Can you work these out from the model? Positions are in its coordinate system, mm. Give positions to 0.01 mm unless a question says otherwise; leave off trailing zeros. Order: outer loops, then holes, each group sorted by start corner. A loop starts at its lowest first (then second) coordinate and runs counter-clockwise, first axis right, second up. Notation, with made-up numbers: (66, -36) - (110, -36) arc R36 cw to (110, 3) - close; hole circle Ø9 at (61, 58.5). An arc over 180 degrees is marked (long way). Answer as a JSON object with one key per item and string values.
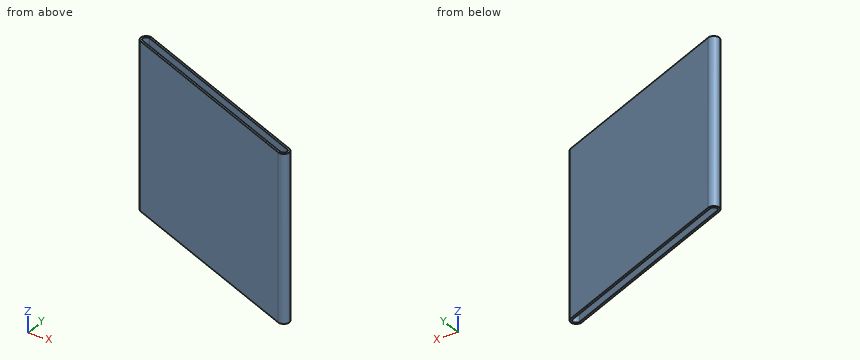
```python
from build123d import *

# Parameters (mm, degrees)
BOSS_EXTRUDE1_DEPTH = 304.8


with BuildPart() as part:
    # Sketch1 → Boss-Extrude1 (new body)
    with BuildSketch(Plane.XY):
        Polygon((-349.09639238, 167.575084446), (6.50360762, 15.175084446), (8.004440147, 18.67702701), (-347.595559853, 171.07702701), align=None)
        Polygon((-354.099167472, 155.901942564), (1.500832528, 3.501942564), (0, 0), (-355.6, 152.4), align=None)
        with BuildLine():
            ThreePointArc((-349.09639238, 167.575084446), (-357.434350867, 164.239901051), (-354.099167472, 155.901942564))
            Line((-354.099167472, 155.901942564), (-355.6, 152.4))
            ThreePointArc((-355.6, 152.4), (-360.936293431, 165.740733579), (-347.595559853, 171.07702701))
            Line((-347.595559853, 171.07702701), (-349.09639238, 167.575084446))
        make_face()
        with BuildLine():
            ThreePointArc((1.500832528, 3.501942564), (9.838791014, 6.837125959), (6.50360762, 15.175084446))
            Line((6.50360762, 15.175084446), (8.004440147, 18.67702701))
            ThreePointArc((8.004440147, 18.67702701), (13.340733579, 5.336293431), (0, 0))
            Line((0, 0), (1.500832528, 3.501942564))
        make_face()
    extrude(amount=BOSS_EXTRUDE1_DEPTH)


solid = part.part
```
Q1. If we section it at B-B, the plane z = 35: Please give me the cut outline in (x, y).
Recorded:
{"outline": "(-355.6, 152.4) - (0, 0) arc R10.16 ccw to (8, 18.68) - (-347.6, 171.08) arc R10.16 ccw to start; hole (-354.1, 155.9) - (1.5, 3.5) arc R6.35 ccw to (6.5, 15.18) - (-349.1, 167.58) arc R6.35 ccw to start"}
Q2. If we section it at C-C, the plane y = 123: Please give me the cut outline in (x, z), then the cut area to 3 significant figures.
Recorded:
{"outline": "(-287, 0) - (-277.33, 0) - (-277.33, 304.8) - (-287, 304.8) - close; (-245.09, 0) - (-235.42, 0) - (-235.42, 304.8) - (-245.09, 304.8) - close", "area": "5,900 mm^2"}
Q3. If we section it at A-A, the plane x = -248.5: Please give me the cut outline in (y, z), then the cut area to 3 significant figures.
Recorded:
{"outline": "(106.5, 0) - (110.65, 0) - (110.65, 304.8) - (106.5, 304.8) - close; (124.46, 0) - (128.61, 0) - (128.61, 304.8) - (124.46, 304.8) - close", "area": "2,530 mm^2"}
Q4. I'm going to push flat-ended pins straight in: pin 1 Ø4 at (x, z) = (-74.5, 65) entering from +Y; pin 2 Ø3 at (x, z) = (-81, 48.5) entering from +Y; pin 3 Ø1.5 at (x, z) = (-131, 255) entering from -Y; pin 4 Ø12 at (x, y) = (-153.5, 65.5) entering from -Z. Where does each tip first touch, or does it pass through?
Recorded:
{"pin 1": "stops at y = 54.89", "pin 2": "stops at y = 57.46", "pin 3": "stops at y = 55.82", "pin 4": "stops at z = 0"}
Q5. I need wall thicknesses on L1, parallel to X at y = 25.5, z = 144; L2, parallel to Y at x = -327, z = 126.5; L3, parallel to X at y = 61, z = 181.5. Which ranges of each line are inside material? Lowest first, please.
Recorded:
{"L1": "x = -59.5 to -49.83, -17.59 to -7.92", "L2": "y = 140.14 to 144.29, 158.11 to 162.25", "L3": "x = -142.33 to -132.66, -100.42 to -90.75"}
